from build123d import *

# Parameters (mm, degrees)
BOSS_EXTRUDE1_DEPTH     = 15
CUT_EXTRUDE1_DEPTH      = 576.044354215
CUT_EXTRUDE1_DEPTH_BACK = 576.044354215
SCALE1_SCALE            = 0.6


with BuildPart() as part:
    # Sketch1 → Boss-Extrude1 (new body)
    with BuildSketch(Plane.XY):
        with BuildLine():
            Line((-236.729376996, 0), (0, 0))
            Line((0, 0), (357.876847169, 0))
            Line((357.876847169, 0), (396.730398779, 416))
            Line((396.730398779, 416), (315.832809595, 416))
            Line((315.832809595, 416), (236.983089551, 242.144494596))
            ThreePointArc((236.983089551, 242.144494596), (164.696190822, 146.877858304), (58.352308735, 92.177707838))
            Line((58.352308735, 92.177707838), (-236.729376996, 16.274880501))
            Line((-236.729376996, 16.274880501), (-236.729376996, 0))
        make_face()
    extrude(amount=BOSS_EXTRUDE1_DEPTH)

    # Sketch2 → Cut-Extrude1 (cut, two sides: drawn at the far end of the back side and taken through both)
    with BuildSketch(Plane.XY.offset(15).offset(-CUT_EXTRUDE1_DEPTH_BACK)):
        Polygon((396.730398779, 416), (357.876847169, 0), (296.597151769, 0), (371.734942748, 416), align=None)
    extrude(amount=CUT_EXTRUDE1_DEPTH + CUT_EXTRUDE1_DEPTH_BACK, mode=Mode.SUBTRACT)


with BuildPart() as part_1:
    # Scale1: scaled about (174.395350586, 126.79859987, 7.5)
    add(part.part.scale(SCALE1_SCALE).moved(Location((69.758140234, 50.719439948, 3))))


solid = part_1.part
CAD build for the part. Positions are in the model's coordinates, mm. Coordinates: 2 decimals unless noted, no trailing zeros. Loops run counter-clockwise (first coordinate to the right, second up) from the corner with the lowest first, then second, coordinate; pieces in that order, holes last. Notation, with made-up numbers: (-15, 23.25) - (0, 23.25) arc R16 cw to (0, 38.25) - close; hole circle Ø4 at (-16.5, 57.25). An arc over 180 degrees is marked (long way). Use one line per item in the form item = value. Start each with the question number.
1) Band-saw the part on C-C (y = 259.5). Give the cut face in (x, z), and give its area (3 significant figures).
2) Band-saw the part on B-B (y = 126). Give the cut face in (x, z).
3) Flat gauge pins, fed straight in: pin 1 (3 mm diameter, centred on x = 227, z = 4.5, fed in from +Y); pin 2 (4 mm diameter, centred on y = 219, z = 8, fed in from +X); pin 3 (4 mm diameter, centred on x = 101, z = 8.5, fed in from +Y). Where does each tip first touch, or does it go through?
4) Band-saw the part on A-A (z = 9.5). Give the cut face in (x, y), and give its area (3 significant figures).
5) Two-plate mould, pull along X, no slides. Class faces 1 (the face through (269.94, 173.77, 7.44)), 2 (the face through (85, 50.719, 7)), 3 (the face through (235.934, 248.893, 7.437)): +X half, -X half, draft (parallel to the pull), parting line (faces both ways), or undercut.
6) Drill centre lines: L1, parallel to Y at x = 189, z = 9; L2, parallel to Y at x = 241.5, z = 7.75; L3, parallel to X at y = 146, z = 6.25. Where is each one in solid material? Low to high. Write a range as from..to.
Check values:
q1.outline = (240.74, 3) - (285.43, 3) - (285.43, 12) - (240.74, 12) - close
q1.area = 402 mm2
q2.outline = (151, 3) - (261.31, 3) - (261.31, 12) - (151, 12) - close
q3.pin_1 = 232.5
q3.pin_2 = 278.47
q3.pin_3 = 105.57
q4.outline = (-72.28, 50.72) - (247.72, 50.72) - (292.8, 300.32) - (259.26, 300.32) - (211.95, 196.01) arc R162 cw to (104.77, 106.03) - (-72.28, 60.48) - close
q4.area = 27,100 mm2
q5.face_1 = +X half
q5.face_2 = draft
q5.face_3 = -X half
q6.L1 = 50.72..159.37
q6.L2 = 50.72..261.17
q6.L3 = 176.55..264.93
